from build123d import *

# Parameters (mm, degrees)
SKETCH1_W               = 152.4
SKETCH1_H               = 50.8
BOSS_EXTRUDE2_DEPTH     = 9.525
CUT_EXTRUDE1_START      = -9.525
CUT_EXTRUDE1_DEPTH      = 9.525
CUT_EXTRUDE2_DEPTH      = 81.884643938
CUT_EXTRUDE2_DEPTH_BACK = 81.884643938


# Read off the part's stored shape, not the designer's step: Cut-Extrude1
with BuildPart() as part:
    # Sketch1 → Boss-Extrude2 (new body)
    with BuildSketch(Plane.XY):
        Rectangle(SKETCH1_W, SKETCH1_H)
    extrude(amount=BOSS_EXTRUDE2_DEPTH)

    # Sketch2 → 1/4-20 Tapped Hole1 (revolve, cut)
    with BuildSketch(Plane(origin=(-25.4, 0, 9.525), x_dir=(0, -1, 0), z_dir=(1, 0, 0))):
        Polygon((0, 0), (0, 9.525), (3.1877, 9.525), (2.5527, 8.89), (2.5527, 0.635), (3.1877, 0), align=None)
    revolve(axis=Axis((-25.4, 0, 15.875), (0, 0, -1)), mode=Mode.SUBTRACT)

    # Cut-Extrude1 outline → Cut-Extrude1 (cut)
    with BuildSketch(Plane.XY.offset(9.525).offset(CUT_EXTRUDE1_START)):
        with BuildLine():
            Line((-76.2, -25.4), (-50.8, -25.4))
            ThreePointArc((-50.8, -25.4), (-68.760512242, -17.960512242), (-76.2, 0))
            Line((-76.2, 0), (-76.2, -25.4))
        make_face()
        with BuildLine():
            Line((-76.2, 25.4), (-76.2, 0))
            ThreePointArc((-76.2, 0), (-68.760512242, 17.960512242), (-50.8, 25.4))
            Line((-50.8, 25.4), (-76.2, 25.4))
        make_face()
    extrude(amount=CUT_EXTRUDE1_DEPTH, mode=Mode.SUBTRACT)

    # Sketch5 → Cut-Extrude2 (cut, two sides: drawn at the far end of the back side and taken through both)
    with BuildSketch(Plane.XY.offset(9.525).offset(-CUT_EXTRUDE2_DEPTH_BACK)):
        Polygon((50.8, -359.042550973), (50.8, -51.798163577), (50.8, 47.427693525), (50.8, 354.672080921), (665.288774792, 354.672080921), (665.288774792, -359.042550973), align=None)
    extrude(amount=CUT_EXTRUDE2_DEPTH + CUT_EXTRUDE2_DEPTH_BACK, mode=Mode.SUBTRACT)


solid = part.part
Verification items for the finished model (mm, model axes). Give positions to 0.01 mm unless a question says otherwise; leave off trailing zeros. Loops run counter-clockwise (first coordinate to the right, second up) from the corner with the lowest first, then second, coordinate; pieces in that order, holes last.
1) Sectioned sample at A-A, the plane x = -25.4. Enter the section's corners in (y, z) (3 decimals), then the cut area to 3 significant figures.
2) Depth check by flat-ended pin: pin 1 Ø2 at (x, z) = (-54, 2) entering from -Y; pin 2 Ø5 at (y, z) = (-14.5, 3.5) entering from -X; pin 3 Ø6 at (x, y) = (-25.4, 0) entering from +Z. Enter the tip coordinate at first touch or a pass-through.
3) Draft check along Y on faces 1 (the flat face through (-1, -25.4, 5)), 2 (the cylindrical face through (-27.552, -1.372, 4.82)), 3 (the flat face through (50.8, 0, 5)). Enter one of: pulls with the +Y half, pulls with the -Y half, needs draft (parallel to the pull), parting line crosses it, or undercut.
4) Sectioned sample at D-D, the plane y = 11. Enter the section's corners in (x, z) (3 decimals).
5) Thickness scan on line 1 along X through (y, z) = (0, 6.5); line 2 along Y through (x, z) = (-25.4, 3.5); line 3 along X through (y, z) = (1.5, 7.5). Record the ranges inside material, lowest first.
6) Sectioned sample at B-B, the plane z = 5. Enter the section's corners in (x, y), then the cut area to 3 significant figures.
7) Sectioned sample at C-C, the plane y = -12.5. Enter the section's corners in (x, z) (3 decimals).
Answers:
1. outline: (-25.4, 0) - (-3.188, 0) - (-2.553, 0.635) - (-2.553, 8.89) - (-3.188, 9.525) - (-25.4, 9.525) - close; (2.553, 0.635) - (3.188, 0) - (25.4, 0) - (25.4, 9.525) - (3.188, 9.525) - (2.553, 8.89) - close
1. area: 434 mm2
2. pin 1: stops at y = -25.3
2. pin 2: stops at x = -73.19
2. pin 3: stops at z = 9.34
3. face 1: pulls with the -Y half
3. face 2: undercut
3. face 3: needs draft
4. outline: (-73.695, 0) - (50.8, 0) - (50.8, 9.525) - (-73.695, 9.525) - close
5. line 1: x = -76.2 to -27.95, -22.85 to 50.8
5. line 2: y = -25.4 to -2.55, 2.55 to 25.4
5. line 3: x = -76.16 to -27.47, -23.33 to 50.8
6. outline: (-50.8, -25.4) - (50.8, -25.4) - (50.8, 25.4) - (-50.8, 25.4) arc R25.4 ccw to start; hole circle Ø5.11 at (-25.4, 0)
6. area: 6,150 mm2
7. outline: (-72.911, 0) - (50.8, 0) - (50.8, 9.525) - (-72.911, 9.525) - close
